Could you check a few things on this model? Use its own coordinates, in mm. A direction names the side the tool comes from. Give positions to 0.01 mm unless a question says otherwise; leave off trailing zeros. Loops run counter-clockwise (first coordinate to the right, second up) from the corner with the lowest first, then second, coordinate; pieces in that order, holes last. Notation, with made-up numbers: (29, -1) -> (60, -1) arc R18 cw to (60, 29) -> close; hole circle Ø2 at (31, 86.5). An arc over 180 degrees is marked (long way). Put each result on its own line as item: value.
Autodesk Inventor part; units mm, degrees
ref_plane "Work Plane1" through (37.5, 0, 0) normal (-1, 0, 0) x (0, 0, 1)
ref_plane "YZ Plane" through (0, 0, 0) normal (1, 0, 0) x (0, 1, 0)
ref_plane "XZ Plane" through (0, 0, 0) normal (0, 1, 0) x (-1, 0, 0)
sketch "Sketch1" plane through (0, 0, 0) normal (0, 0, 1) x (1, 0, 0)
  line L0 (0, 0) -> (75, 0)
  line L1 (75, 0) -> (75, 30)
  line L2 (75, 30) -> (0, 30)
  line L3 (0, 30) -> (0, 0)
  circle A0 centre (17.5, 15) radius 2.5
  circle A1 centre (57.5, 15) radius 2.5
  line L4 (17.5, 15) -> (57.5, 15) construction
  point P0 (37.5, 15)
  point P1 (37.5, 30)
  dimension "d0" = 75
  dimension "d1" = 30
  dimension "d2" = 5
  dimension "d3" = 5
  dimension "d4" = 40
  dimension "d5" = 15
extrude "Extrusion1" add sketch "Sketch1" along normal blind 5
sketch "Sketch2" plane through (75, 0, 0) normal (1, 0, 0) x (0, 0, -1)
  circle A0 centre (-15, -10) radius 4
  circle A1 centre (-15, -10) radius 7.5 construction
  line L0 (-5, 0) -> (-5, 30) construction
  arc A2 (-5, 30) -> (-22.4763, -9.4047) centre (42.3186, -14.564) ccw
  arc A3 (-5, 0) -> (-7.5195, -9.4597) centre (7.4415, -8.379) ccw
  arc A4 (-22.4763, -9.4047) -> (-7.5195, -9.4597) centre (-15, -10) ccw
  line L1 (0, 0) -> (-5, 0)
  line L2 (0, 30) -> (-5, 30)
  line L3 (-5, 30) -> (-5, 0)
  dimension "d8" = 8
  dimension "d9" = 15
  dimension "d10" = 10
  dimension "d11" = 10
  dimension "d12" = 65
  dimension "d13" = 15
extrude "Extrusion2" add sketch "Sketch2" against normal blind 10
sketch "Sketch3" plane through (0, 0, 0) normal (-1, 0, 0) x (0, 0, 1)
  circle A0 centre (15, -10) radius 4
  arc A1 (7.5195, -9.4597) -> (5, 0) centre (-7.4415, -8.379) ccw
  arc A2 (7.5195, -9.4597) -> (22.4763, -9.4047) centre (15, -10) ccw
  arc A3 (22.4763, -9.4047) -> (5, 30) centre (-42.3186, -14.564) ccw
  line L0 (5, 0) -> (5, 30)
  point P0 (0, 0)
extrude "Extrusion3" add sketch "Sketch3" against normal blind 10
ref_plane "Work Plane1" through (37.5, 0, 0) normal (-1, 0, 0) x (0, 0, 1)
sketch "Sketch4" plane through (37.5, 0, 0) normal (-1, 0, 0) x (0, 0, 1)
  circle A0 centre (15, -10) radius 4
  arc A1 (7.5195, -9.4597) -> (5, 0) centre (-7.4415, -8.379) ccw
  arc A2 (7.5195, -9.4597) -> (22.4763, -9.4047) centre (15, -10) ccw
  arc A3 (22.4763, -9.4047) -> (5, 30) centre (-42.3186, -14.564) ccw
  line L0 (5, 0) -> (5, 30)
  point P0 (0, 0)
extrude "Extrusion4" add sketch "Sketch4" along normal mid plane 20
sketch "Sketch5" plane through (0, 0, 5) normal (0, 0, 1) x (1, 0, 0)
  circle A0 centre (17.5, 15) radius 2.5
  line L0 (27.5, 0) -> (27.5, 30)
  line L1 (27.5, 30) -> (10, 30)
  line L2 (10, 30) -> (10, 0)
  line L3 (10, 0) -> (27.5, 0)
  line L4 (47.5, 30) -> (47.5, 0)
  line L5 (47.5, 0) -> (65, 0)
  line L6 (65, 0) -> (65, 30)
  line L7 (65, 30) -> (47.5, 30)
  circle A1 centre (57.5, 15) radius 2.5
  point P0 (0, 0)
extrude "Extrusion5" add sketch "Sketch5" along normal blind 5
sketch "Sketch6" plane through (75, 0, 0) normal (1, 0, 0) x (0, 0, -1)
  line L0 (0, 0) -> (-5, 0)
  line L1 (0, 30) -> (-5, 30)
  line L2 (0, 0) -> (-5, 0)
  line L3 (-5, 0) -> (-5, 30)
  line L4 (-5, 30) -> (0, 30)
  line L5 (0, 30) -> (0, 0)
  arc A0 (-5, 30) -> (-10, 24.0076) centre (42.3186, -14.564) ccw
  line L6 (-5, 30) -> (-10, 30)
  line L7 (-10, 24.0076) -> (-10, 30)
extrude "Extrusion6" cut sketch "Sketch6" against normal through all
sketch "Sketch7" plane through (0, 0, 5) normal (-1, 0, 0) x (0, 0, 1)
  circle A0 centre (10, -10) radius 4
  point P0 (-5, 0)
extrude "Extrusion7" add sketch "Sketch7" against normal blind 11
sketch "Sketch8" plane through (27.5, 0, 0) normal (-1, 0, 0) x (0, 0, 1)
  line L0 (10, 24.0076) -> (10, 0)
  line L1 (10, 0) -> (5, 0)
  arc A0 (7.5195, -9.4597) -> (5, 0) centre (-7.4415, -8.379) ccw
  arc A1 (7.5195, -9.4597) -> (22.4763, -9.4047) centre (15, -10) ccw
  arc A2 (22.4763, -9.4047) -> (10, 24.0076) centre (-42.3186, -14.564) ccw
  circle A3 centre (15, -10) radius 4
  point P0 (0, 0)
extrude "Extrusion8" add sketch "Sketch8" along normal blind 1 and the other way blind 21 contours A3
sketch "Sketch9" plane through (75, 0, 5) normal (1, 0, 0) x (0, 0, -1)
  circle A0 centre (-10, -10) radius 4
  point P0 (5, 0)
extrude "Extrusion9" add sketch "Sketch9" against normal blind 11
fillet "Fillet1" radius 1 4 edges at (11, -10, 11) (26.5, -10, 11) (48.5, -10, 11) (64, -10, 19)
properties part number "TC006b" material "ABS Plastic"
1. If we section it at D-D (x = 67): List the corners of the cut face in (y, z) for me, then the cut area to 3 significant figures.
Recorded:
outline: (-9.46, 7.52) arc R15 cw to (0, 5) -> (30, 5) arc R65 ccw to (-9.4, 22.48) arc R7.5 ccw (long way) to start
area: 531 mm^2
2. I need wall thicknesses on line 1 (X direction, y = 15, z = 7.95); line 2 (X direction, y = -8, z = 21); line 3 (Y direction, x = 17.5, z = 8.85). Which ranges of each line are inside material? Lowest first, please.
Recorded:
line 1: x = 0 to 15, 20 to 55, 60 to 75
line 2: x = 0 to 10, 27.5 to 47.5, 65 to 75
line 3: y = 0 to 12.5, 17.5 to 25.52
3. If we section it at B-B (z = 21.5): List the corners of the cut face in (x, y) for me.
Recorded:
outline: (0, -13.74) -> (10, -13.74) -> (10, -2.23) -> (0, -2.23) -> close; (27.5, -13.74) -> (47.5, -13.74) -> (47.5, -2.23) -> (27.5, -2.23) -> close; (65, -13.74) -> (75, -13.74) -> (75, -2.23) -> (65, -2.23) -> close
4. If we section it at C-C (y = 15): List the corners of the cut face in (x, z) for me, then the cut area to 3 significant figures.
Recorded:
outline: (0, 5) -> (15, 5) -> (15, 10) -> (10, 10) -> (10, 15.57) -> (0, 15.57) -> close; (20, 5) -> (55, 5) -> (55, 10) -> (47.5, 10) -> (47.5, 15.57) -> (27.5, 15.57) -> (27.5, 10) -> (20, 10) -> close; (60, 5) -> (75, 5) -> (75, 15.57) -> (65, 15.57) -> (65, 10) -> (60, 10) -> close
area: 548 mm^2
5. I'm going to push flat-ended pins straight in: pin 1 (4.5 mm diameter, centred on x = 17.5, y = 15, fed in from +Z); pin 2 (6 mm diameter, centred on x = 57.5, y = 15, fed in from +Z); pin 3 (8 mm diameter, centred on x = 48, y = 4.5, fed in from +Z); pin 4 (1 mm diameter, centred on x = 19.5, z = 9, fed in from -Y). Where does each tip first touch, or does it pass through?
Recorded:
pin 1: passes through
pin 2: stops at z = 10
pin 3: stops at z = 20.9
pin 4: stops at y = 0
6. If we section it at A-A (x = 57.5): List the corners of the cut face in (y, z) for me.
Recorded:
outline: (0, 5) -> (12.5, 5) -> (12.5, 10) -> (0, 10) -> close; (17.5, 5) -> (30, 5) arc R65.01 ccw to (24.01, 10) -> (17.5, 10) -> close
7. For faces 1 (the face through (48.5, -10, 15)), 2 (the face through (37.64, -4.451, 7.035)), 3 (the face through (70.07, 12.069, 16.974)), which set-ups out of +Z, -Z, +X, -X, +Y, -Y let a thin tool reach every point of the face, with its end or its side?
Recorded:
face 1: +Z, -Z, +Y, -Y
face 2: -Z, +X, -X
face 3: +Z, +X, -X, +Y
8. Thinking about a two-plate mould opening in X: for faces 4 (the face through (0, 1, 12)), 5 (the face through (64, -10, 15)), 6 (the face through (18.873, 27.121, 7.555)), which applies, pulls with the +X half, pulls with the -X half, needs draft (parallel to the pull), parting line crosses it, or undercut?
Recorded:
face 4: pulls with the -X half
face 5: undercut
face 6: needs draft
